Autodesk Inventor part; units mm, degrees
ref_plane "YZ Plane" through (0, 0, 0) normal (1, 0, 0) x (0, 1, 0)
ref_plane "XZ Plane" through (0, 0, 0) normal (0, 1, 0) x (-1, 0, 0)
ref_plane "XY Plane" through (0, 0, 0) normal (0, 0, 1) x (1, 0, 0)
sketch "Sketch1" plane through (0, 0, 0) normal (0, 0, 1) x (1, 0, 0)
  line L0 (-25, -26) -> (25, -26)
  line L1 (25, -26) -> (25, 26)
  line L2 (25, 26) -> (-25, 26)
  line L3 (-25, 26) -> (-25, -26)
  line L4 (-25, -26) -> (25, 26) construction
  line L5 (25, -26) -> (-25, 26) construction
  circle A0 centre (0, 2) radius 8.8
  circle A1 centre (-14.5, 2) radius 2.25
  circle A2 centre (14.5, 2) radius 2.25
  point P0 (0, 0)
  dimension "d0" = 50
  dimension "d1" = 52
  dimension "d2" = 17.6
  dimension "d3" = 24
  dimension "d4" = 4.5
  dimension "d5" = 4.5
  dimension "d6" = 29
  dimension "d7" = 14.5
  dimension "d8" = 24
  dimension "d9" = 24
  dimension "d10" = 25
extrude "Plate1" add sketch "Sketch1" along normal blind 3
sketch "Sketch2" plane through (25, -23, 0) normal (0, -1, 0) x (1, 0, 0)
  line L0 (-50, 0) -> (0, 0)
  line L1 (0, 0) -> (0, 52)
  line L2 (0, 52) -> (-50, 52)
  line L3 (-50, 52) -> (-50, 0)
edge flange "Flange1" height 52 angle 90 thickness 3 bend radius 3 thickness toward (0, -1, 0) relief tear relief width 3 relief depth 1.5 edges at (0, -26, 3) wall of the first edge with corners at (-25, -23, 0) (25, -23, 0) (25, -23, 52) (-25, -23, 52)
bend "Bend1"
corner "Corner1"
fillet "Fillet1" radius 10 2 edges at (25, 26, 1.5) (-25, 26, 1.5)
fillet "Fillet2" radius 5 2 edges at (-25, -24.5, 52) (25, -24.5, 52)
sketch "Sketch3" plane through (-25, -26, 6) normal (0, -1, 0) x (1, 0, 0)
  line L0 (8.5, 38.5) -> (41.5, 38.5)
  line L1 (41.5, 38.5) -> (41.5, 5.5)
  line L2 (41.5, 5.5) -> (8.5, 5.5)
  line L3 (8.5, 5.5) -> (8.5, 38.5)
  line L4 (8.5, 38.5) -> (41.5, 5.5) construction
  line L5 (41.5, 38.5) -> (8.5, 5.5) construction
  line L6 (5, 46) -> (45, 46)
  line L7 (50, 41) -> (50, 0)
  circle A0 centre (41.5, 38.5) radius 2.25
  circle A1 centre (41.5, 5.5) radius 2.25
  circle A2 centre (8.5, 38.5) radius 2.25
  circle A3 centre (8.5, 5.5) radius 2.25
  point P0 (25, -6)
  point P1 (25, 22)
  dimension "d24" = 33
  dimension "d25" = 33
  dimension "d26" = 24
  dimension "d27" = 25
  dimension "d28" = 4.5
  dimension "d29" = 4.5
  dimension "d30" = 4.5
  dimension "d31" = 4.5
extrude "Cut1" cut sketch "Sketch3" against normal blind 3 contours L3 A2 L0 | L0 A2 L3 | A0 L1 L0 | L0 L1 A0 | A3 L2 L3 | L3 L2 A3 | A1 L2 L1 | L1 L2 A1
equation "\"d32\" = Thickness"
equation "\"d11\" = Thickness"
equation "\"d12\" = BendReliefWidth"
equation "\"d13\" = BendReliefDepth"
equation "\"d14\" = MinimumRemnant"
equation "\"d15\" = TransitionRadius"
equation "\"d18\" = BendRadius"
equation "\"d19\" = CornerReliefSize"
equation "\"d20\" = GapSize"
equation "\"d21\" = JacobiRadiusSize"
equation "\"BendRadius\" = Thickness"
equation "\"BendReliefWidth\" = Thickness"
equation "\"BendReliefDepth\" = 0.5 * Thickness"
equation "\"CornerReliefSize\" = 4 * Thickness"
equation "\"MinimumRemnant\" = 2 * Thickness"
equation "\"TransitionRadius\" = BendRadius"
equation "\"JacobiRadiusSize\" = BendRadius"
equation "\"GapSize\" = Thickness"
properties part number "Pad dong co 775"
Read the model definition and answer for the solid it produces. Units are mm, in the model's axes. A direction names the side the tool comes from. Give positions to 0.01 mm unless a question says otherwise; leave off trailing zeros. Loops run counter-clockwise (first coordinate to the right, second up) from the corner with the lowest first, then second, coordinate; pieces in that order, holes last.
Item 1: The mould has two halves that part along Z. Classify faces 3 (the cylindrical face through (-16.79, -24.52, 46.73)), 4 (the cylindrical face through (0.35, -24.289, 1.804)), 5 (the flat face through (0, -26, 29)): released by +Z, released by -Z, zero draft, split by the parting line, or undercut.
Item 2: The part is cut by section B-B (y = 2). Write down the section's boundary in (x, z), and give its area (3 significant figures).
Item 3: For faces 1 (the flat face through (0, -7, 3)), 2 (the cylindrical face through (17.71, -24.521, 13.397)), determine the directions among +Z, -Z, +X, -X, +Y, -Y from which every point of the face is accessible in a straight line to the end or side of a thin tool.
Item 4: Find the intervals of material crossed by line 1 along X through (y, z) = (-24.5, 11.5); line 2 along Y through (x, z) = (23, 30.5); line 3 along Z through (x, y) = (15, 21), in increasing order.
Item 5: The part is cut by section D-D (x = 18). Write down the section's boundary in (y, z), and give its area (3 significant figures).
Item 6: The part is cut by section C-C (z = 11.5). Write down the section's boundary in (x, y), and give its area (3 significant figures).
Item 7: Each of these flat-tipped pins is pushed along its axis until it touches: pin 1 Ø5 at (x, y) = (-14.5, 2) entering from +Z; pin 2 Ø7 at (x, z) = (-16.5, 44.5) entering from +Y; pin 3 Ø6 at (x, z) = (16.5, 11.5) entering from -Y; pin 4 Ø3 at (x, z) = (12, 6.5) entering from +Y. Where does it stop, or does it pass through?
Item 8: The part is cut by section A-A (x = 0). Write down the section's boundary in (y, z), and give its area (3 significant figures).
Taken from the geometry:
1. face 3: undercut
1. face 4: released by -Z
1. face 5: zero draft
2. outline: (-25, 0) - (-16.75, 0) - (-16.75, 3) - (-25, 3) - close; (-12.25, 0) - (-8.8, 0) - (-8.8, 3) - (-12.25, 3) - close; (8.8, 0) - (12.25, 0) - (12.25, 3) - (8.8, 3) - close; (16.75, 0) - (25, 0) - (25, 3) - (16.75, 3) - close
2. area: 70.2 mm2
3. face 1: +Z, +X, -X, +Y
3. face 2: +Y, -Y
4. line 1: x = -25 to -18.75, -14.25 to 14.25, 18.75 to 25
4. line 2: y = -26 to -23
4. line 3: z = 0 to 3
5. outline: (-26, 6) arc R6 ccw to (-20, 0) - (25.54, 0) - (25.54, 3) - (-20, 3) arc R3 cw to (-23, 6) - (-23, 9.82) - (-26, 9.82) - close; (-26, 13.18) - (-23, 13.18) - (-23, 42.82) - (-26, 42.82) - close; (-26, 46.18) - (-23, 46.18) - (-23, 52) - (-26, 52) - close
5. area: 276 mm2
6. outline: (-25, -26) - (-18.75, -26) - (-18.75, -23) - (-25, -23) - close; (-14.25, -26) - (14.25, -26) - (14.25, -23) - (-14.25, -23) - close; (18.75, -26) - (25, -26) - (25, -23) - (18.75, -23) - close
6. area: 123 mm2
7. pin 1: stops at z = 3
7. pin 2: stops at y = -23
7. pin 3: stops at y = -26
7. pin 4: stops at y = -22.83
8. outline: (-26, 6) arc R6 ccw to (-20, 0) - (-6.8, 0) - (-6.8, 3) - (-20, 3) arc R3 cw to (-23, 6) - (-23, 52) - (-26, 52) - close; (10.8, 0) - (26, 0) - (26, 3) - (10.8, 3) - close
8. area: 244 mm2
